Verification items for this drawing (mm, ordinates from the low corner). A direction names the side the tool comes from. Round coordinates to 2 decimals unless told otherwise and drop trailing zeros. Loops run counter-clockwise (first coordinate to the right, second up) from the corner with the lowest first, then second, coordinate; pieces in that order, holes last. Notation, with made-up numbers: (53.25, -1.5) -> (95.25, -1.5) arc R17 ccw to (95.25, 10.5) -> close; hole circle Ø4 at (-23.75, -16). An arc over 180 degrees is marked (long way). Use a Markdown table: item, result. Add a question column.
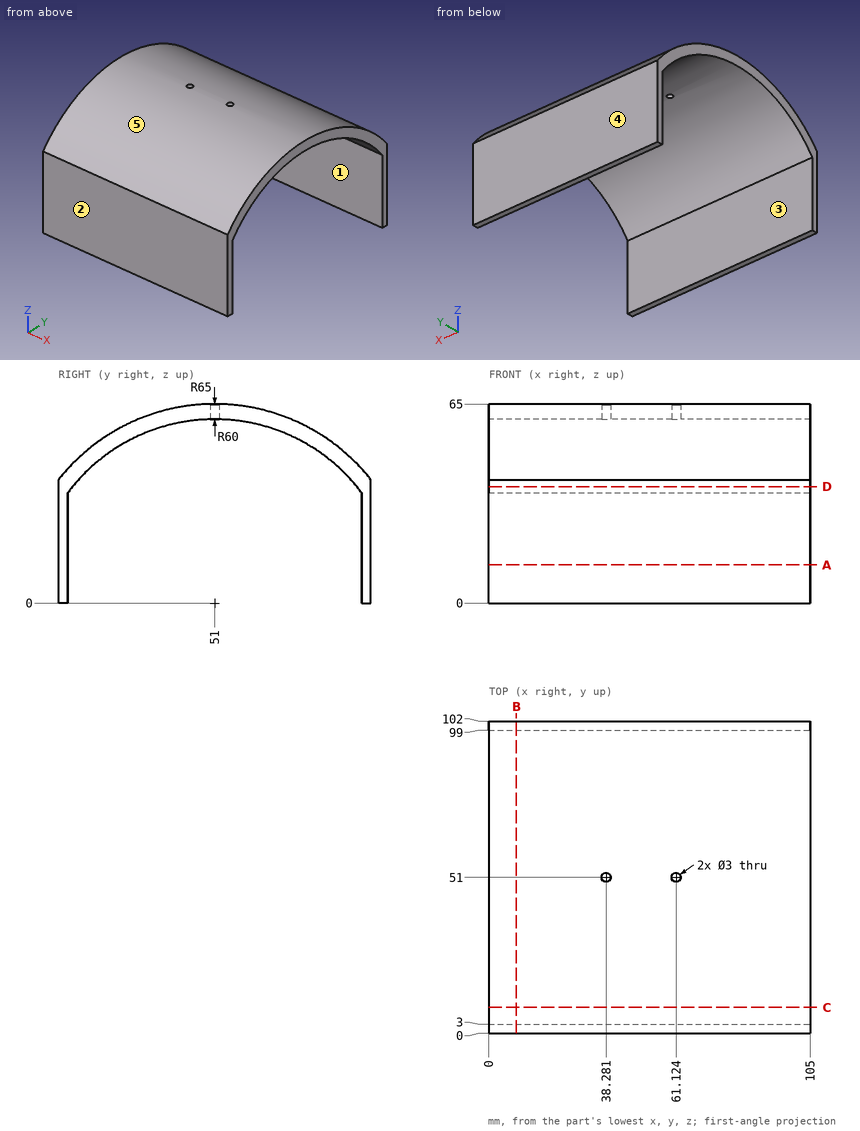
1) Go/stop test with flat-tipped pins: pin 1 (8 mm diameter, centred on x = 72.5, y = 14.5, fed in from +Z); pin 2 (1.5 mm diameter, centred on x = 55, y = 87.5, fed in from +Z) (1 decimal); pin 3 (1.5 mm diameter, centred on x = 30.5, z = 45.5, fed in from -Y); pin 4 (2.5 mm diameter, centred on x = 61.12, y = 51, fed in from +Z). Record where each tip stops, or that it passes through.
2) Sectioned sample at A-A on z = 12.5. Enter the section's corners in (x, y), then the cut area to 3 significant figures.
3) Sectioned sample at B-B on x = 9. Enter the section's corners in (y, z).
4) Thickness scan on line 1 (X direction, y = 51, z = 62.05) (1 decimal); line 2 (Y direction, x = 91.5, z = 8); line 3 (Y direction, x = 25.5, z = 50) (1 decimal). Record the ranges inside material, lowest first.
5) Release check for a two-part mould opening along Y. For the marked faces 3, 4 and 5 record: released by +Y, released by -Y, zero draft, split by the parting line, or undercut.
6) Access from +Z, -Z, +X, -X, +Y, -Y to the whole of each face (thin tool, end or side, straight path). Record for the marked faces 1 and 2.
7) Sectioned sample at D-D on z = 38. Enter the section's corners in (x, y).
8) Sectioned sample at C-C on y = 8.5. Enter the section's corners in (x, z), then the cut area to 3 significant figures.
Geometry results:
| question | item | result |
|---|---|---|
| 1 | pin 1 | z = 56.29 |
| 1 | pin 2 | z = 54.3 |
| 1 | pin 3 | y = 3.86 |
| 1 | pin 4 | through |
| 2 | outline | (0, 0) -> (105, 0) -> (105, 3) -> (0, 3) -> close; (0, 99) -> (105, 99) -> (105, 102) -> (0, 102) -> close |
| 2 | area | 630 mm^2 |
| 3 | outline | (0, 0) -> (3, 0) -> (3, 36) arc R60 cw to (99, 36) -> (99, 0) -> (102, 0) -> (102, 40.3) arc R65 ccw to (0, 40.3) -> close |
| 4 | line 1 | 0 to 36.8, 39.8 to 59.6, 62.6 to 105 |
| 4 | line 2 | 0 to 3, 99 to 102 |
| 4 | line 3 | 9.5 to 17.8, 84.2 to 92.5 |
| 5 | face 3 | undercut |
| 5 | face 4 | released by +Y |
| 5 | face 5 | split by the parting line |
| 6 | face 1 | -Z, +X, -X |
| 6 | face 2 | +Z, -Z, +X, -X, -Y |
| 7 | outline | (0, 0) -> (105, 0) -> (105, 4.57) -> (0, 4.57) -> close; (0, 97.43) -> (105, 97.43) -> (105, 102) -> (0, 102) -> close |
| 8 | outline | (0, 42.35) -> (105, 42.35) -> (105, 49.18) -> (0, 49.18) -> close |
| 8 | area | 717 mm^2 |
